from build123d import *

# Parameters (mm, degrees)
SKETCH001_W   = 110
SKETCH001_H   = 78
PAD_DEPTH     = 1.6
SKETCH009_R   = 1.5
PAD001_DEPTH  = 6.5
SKETCH010_W   = 110
SKETCH010_H   = 61
PAD002_DEPTH  = 1.2
SKETCH011_W   = 105.6
SKETCH011_H   = 63
PAD003_DEPTH  = 3.8
SKETCH012_W   = 94
SKETCH012_H   = 57
POCKET_DEPTH  = 0.2
SKETCH013_W   = 9
SKETCH013_H   = 6.4
SKETCH013_W_2 = 6.4
SKETCH013_H_2 = 9
PAD004_DEPTH  = 3
SKETCH014_W   = 15
SKETCH014_H   = 14.5
PAD005_DEPTH  = 1.8
SKETCH015_W   = 11
SKETCH015_H   = 0.9
PAD006_DEPTH  = 5.4
SKETCH016_W   = 2.7
SKETCH016_H   = 6.8
SKETCH016_W_2 = 2.6
SKETCH016_H_2 = 4
PAD007_DEPTH  = 1.6
SKETCH017_W   = 1.3
SKETCH017_H   = 1
PAD008_DEPTH  = 1.5
SKETCH018_W   = 11.8
SKETCH018_H   = 11.8
PAD009_DEPTH  = 4
SKETCH019_R   = 3.3
PAD010_DEPTH  = 3.6
SKETCH020_W   = 91
SKETCH020_H   = 66
PAD011_DEPTH  = 5.8


with BuildPart() as part:
    # Sketch001 → Pad (new body)
    with BuildSketch(Plane.XY):
        with Locations((0, -8.5)):
            Rectangle(SKETCH001_W, SKETCH001_H)
    extrude(amount=PAD_DEPTH)

    # Sketch009 (on Face6 of Pad) → Pad001 (join)
    with BuildSketch(Plane.XY.offset(1.6)):
        with Locations((-52.2, 27.7)):
            Circle(SKETCH009_R)
        with Locations((-52.2, -27.7)):
            Circle(SKETCH009_R)
        with Locations((52.2, -27.7)):
            Circle(SKETCH009_R)
        with Locations((52.2, 27.7)):
            Circle(SKETCH009_R)
    extrude(amount=PAD001_DEPTH)

    # Sketch010 (on Face12 of Pad001) → Pad002 (join)
    with BuildSketch(Plane.XY.offset(8.1)):
        Rectangle(SKETCH010_W, SKETCH010_H)
    extrude(amount=PAD002_DEPTH)

    # Sketch011 (on Face5 of Pad002) → Pad003 (join)
    with BuildSketch(Plane.XY.offset(9.3)):
        with Locations((-1.7, 0)):
            Rectangle(SKETCH011_W, SKETCH011_H)
    extrude(amount=PAD003_DEPTH)

    # Sketch012 (on Face19 of Pad003) → Pocket (cut)
    with BuildSketch(Plane.XY.offset(13.1)):
        with Locations((0.9, 0)):
            Rectangle(SKETCH012_W, SKETCH012_H)
    extrude(amount=-POCKET_DEPTH, mode=Mode.SUBTRACT)

    # Sketch013 (on Face4 of Pocket) → Pad004 (join)
    with BuildSketch(Plane(origin=(0, 0, 8.1), x_dir=(1, 0, 0), z_dir=(0, 0, -1))):
        with Locations((-18.9, 27.3)):
            Rectangle(SKETCH013_W, SKETCH013_H)
        with Locations((51.8, 13)):
            Rectangle(SKETCH013_W_2, SKETCH013_H_2)
    extrude(amount=PAD004_DEPTH)

    # Sketch014 (on Face4 of Pad004) → Pad005 (join)
    with BuildSketch(Plane(origin=(0, 0, 8.1), x_dir=(1, 0, 0), z_dir=(0, 0, -1))):
        with Locations((38.9, -23.25)):
            Rectangle(SKETCH014_W, SKETCH014_H)
    extrude(amount=PAD005_DEPTH)

    # Sketch015 (on Face5 of Pad005) → Pad006 (join)
    with BuildSketch(Plane(origin=(0, 30.5, 0), x_dir=(-1, 0, 0), z_dir=(0, 1, 0))):
        with Locations((-37.9, 7.15)):
            Rectangle(SKETCH015_W, SKETCH015_H)
    extrude(amount=PAD006_DEPTH)

    # Sketch016 (on Face4 of Pad006) → Pad007 (join)
    with BuildSketch(Plane(origin=(0, 0, 8.1), x_dir=(1, 0, 0), z_dir=(0, 0, -1))):
        with Locations((53.35, 1.3)):
            Rectangle(SKETCH016_W, SKETCH016_H)
        with Locations((53.7, -6.5)):
            Rectangle(SKETCH016_W_2, SKETCH016_H_2)
        with Locations((53.7, -18.5)):
            Rectangle(SKETCH016_W_2, SKETCH016_H_2)
    extrude(amount=PAD007_DEPTH)

    # Sketch017 (on Face31 of Pad007) → Pad008 (join)
    with BuildSketch(Plane.YZ.offset(54.7)):
        with Locations((-2.15, 7.2)):
            Rectangle(SKETCH017_W, SKETCH017_H)
        with Locations((-0.45, 7.2)):
            Rectangle(SKETCH017_W, SKETCH017_H)
    extrude(amount=PAD008_DEPTH)

    # Sketch018 (on Face50 of Pad008) → Pad009 (join)
    with BuildSketch(Plane.XY.offset(1.6)):
        with Locations((-4.6, -39.7)):
            Rectangle(SKETCH018_W, SKETCH018_H)
        with Locations((-32.7, -39.7)):
            Rectangle(SKETCH018_W, SKETCH018_H)
        with Locations((-46.5, -39.7)):
            Rectangle(SKETCH018_W, SKETCH018_H)
    extrude(amount=PAD009_DEPTH)

    # Sketch019 (on Face87 of Pad009) → Pad010 (join)
    with BuildSketch(Plane.XY.offset(5.6)):
        with Locations((-46.5, -39.7)):
            Circle(SKETCH019_R)
        with Locations((-32.7, -39.7)):
            Circle(SKETCH019_R)
        with Locations((-4.6, -39.7)):
            Circle(SKETCH019_R)
    extrude(amount=PAD010_DEPTH)

    # Sketch020 (on Face85 of Pad010) → Pad011 (join)
    with BuildSketch(Plane(origin=(0, 0, 0), x_dir=(1, 0, 0), z_dir=(0, 0, -1))):
        with Locations((0, 8)):
            Rectangle(SKETCH020_W, SKETCH020_H)
    extrude(amount=PAD011_DEPTH)


with BuildPart() as part_1:
    # Body001 placement: moved
    add(part.part.moved(Location((0, 0, 8.5))))


solid = part_1.part
For this review, take the finished solid that the model builds, in its own axes (mm). A direction names the side the tool comes from. Round coordinates to 2 decimals unless told otherwise and drop trailing zeros. Write each loop counter-clockwise with the first axis right and the second up, starting at its lowest first coordinate (ties: lowest second). Pieces come first, ordered by that corner, then holes. Notation, with made-up numbers: (-7.75, -26) - (30.25, -26) arc R21 ccw to (30.25, 9) - close; hole circle Ø4 at (32.5, 60). An arc over 180 degrees is marked (long way). Write item = value, one per line. Start each with the question number.
1. Consider section D-D on x = 12.5. State the section outline as (y, z) points, plus the area to 3 significant figures.
2. Draft analysis for pull direction Y (two halves, no side actions). For faces 1 (the face through (-33, -45.6, 12)), 2 (the face through (54, 18, 15)), 3 (the face through (-5, -40, 17.7)), state which applies: released by +Y, released by -Y, zero draft, split by the parting line, or undercut.
3. Wall thickness on L1, parallel to Z at x = -21.5, y = -28; L2, parallel to Z at x = 42, y = -3; L3, parallel to X at y = 1.5, z = 9: over which ranges is each line inside the solid? List them lowest first.
4. Consider section A-A on x = -4.6. State the section outline as (y, z) points, plus the area to 3 significant figures.
5. For faces 4 (the face through (45.5, -8, 6)), 5 (the face through (-14.4, -27, 15)), 6 (the face through (52, -13, 13.6)), 7 (the face through (-47, -45.6, 12)), 8 (the face through (0, 0, 21.4)), list the 3-axis set-ups (+Z, -Z, +X, -X, +Y, -Y) from which the entire face can be reached by the end or side of a thin tool; tool diameter is ignored.
6. For pin 1 Ø6.5 at (x, z) = (-18.5, 6) entering from +Y; pin 2 Ø0.8 at (x, z) = (55.5, 15.5) entering from +Y; pin 3 Ø5 at (x, y) = (18, -19) entering from +Z, all flat-tipped, find the tip position at first contact; note any pin that passes through.
7. Consider section B-B on y = -15.5. State the section outline as (x, z) points, plus the area to 3 significant figures.
Evaluation:
q1.outline = (-47.5, 8.5) - (-41, 8.5) - (-41, 2.7) - (25, 2.7) - (25, 8.5) - (30.5, 8.5) - (30.5, 10.1) - (-47.5, 10.1) - close; (-31.5, 17.8) - (-30.5, 17.8) - (-30.5, 16.6) - (30.5, 16.6) - (30.5, 17.8) - (31.5, 17.8) - (31.5, 21.6) - (28.5, 21.6) - (28.5, 21.4) - (-28.5, 21.4) - (-28.5, 21.6) - (-31.5, 21.6) - close
q1.area = 809 mm2
q2.face_1 = released by -Y
q2.face_2 = undercut
q2.face_3 = zero draft
q3.L1 = 2.7 to 10.1, 13.6 to 21.4
q3.L2 = 2.7 to 10.1, 16.6 to 21.4
q3.L3 = -55 to 55
q4.outline = (-47.5, 8.5) - (-41, 8.5) - (-41, 2.7) - (25, 2.7) - (25, 8.5) - (30.5, 8.5) - (30.5, 10.1) - (-33.8, 10.1) - (-33.8, 14.1) - (-36.4, 14.1) - (-36.4, 17.7) - (-43, 17.7) - (-43, 14.1) - (-45.6, 14.1) - (-45.6, 10.1) - (-47.5, 10.1) - close; (-31.5, 17.8) - (-30.5, 17.8) - (-30.5, 16.6) - (30.5, 16.6) - (30.5, 17.8) - (31.5, 17.8) - (31.5, 21.6) - (28.5, 21.6) - (28.5, 21.4) - (-28.5, 21.4) - (-28.5, 21.6) - (-31.5, 21.6) - close
q4.area = 880 mm2
q5.face_4 = -Z, +X, +Y, -Y
q5.face_5 = +Y, -Y
q5.face_6 = +X, -X
q5.face_7 = +Z, +X, -X, -Y
q5.face_8 = +Z
q6.pin_1 = 30.5
q6.pin_2 = 0.2
q6.pin_3 = 21.4
q7.outline = (-55, 8.5) - (-45.5, 8.5) - (-45.5, 2.7) - (45.5, 2.7) - (45.5, 8.5) - (55, 8.5) - (55, 10.1) - (-55, 10.1) - close; (-55, 16.6) - (48.6, 16.6) - (48.6, 13.6) - (55, 13.6) - (55, 17.8) - (51.1, 17.8) - (51.1, 21.6) - (47.9, 21.6) - (47.9, 21.4) - (-46.1, 21.4) - (-46.1, 21.6) - (-54.5, 21.6) - (-54.5, 17.8) - (-55, 17.8) - close
q7.area = 1,240 mm2
